Answer from the drawing. Dimensions are ordinates in mm from the lowest x, y and z of the part. A direction names the side the tool comes from. Give positions to 0.01 mm unless a question says otherwise; leave off trailing zeros. Write each loop counter-clockwise with the first axis right and the second up, starting at its lowest first coordinate (ties: lowest second). Pieces come first, ordered by that corner, then holes. Notation, with made-up numbers: (-16, -23.5) -> (42, -23.5) arc R21 cw to (42, -10.5) -> close; hole circle Ø10 at (37.25, 74.5). An arc over 180 degrees is marked (long way). Put each result on its own line as item: value. Start each with the question number.
1) Find the intervals of material crossed by line 1 along Z through (x, y) = (6.5, 4.75); line 2 along X through (y, z) = (7.5, 3.75); line 3 along Z through (x, y) = (5.5, 10.5), in increasing order. Write a range as from..to.
2) A cutting plane is placed at B-B (x = 11). Write down the section's boundary in (y, z), then the cut area to 3 significant figures.
3) For the marked faces 1, 2 and 3, determine the directions among +Z, -Z, +X, -X, +Y, -Y from which every point of the face is accessible in a straight line to the end or side of a thin tool.
4) A cutting plane is placed at D-D (x = 16.25). Write down the section's boundary in (y, z).
5) A cutting plane is placed at C-C (z = 2.25). Write down the section's boundary in (x, y), then the cut area to 3 significant figures.
6) A cutting plane is placed at A-A (y = 11). Write down the section's boundary in (x, z), then the cut area to 4 significant figures.
7) Flat-ended cylindrical pins translate along their axes: pin 1 Ø12 at (y, z) = (6, 7.5) entering from -X; pin 2 Ø3 at (y, z) = (9.5, 16.5) entering from +X; pin 3 Ø8 at (y, z) = (6.5, 6.5) entering from +X. Find the tip coordinate at first contact, or state that the pin passes through.
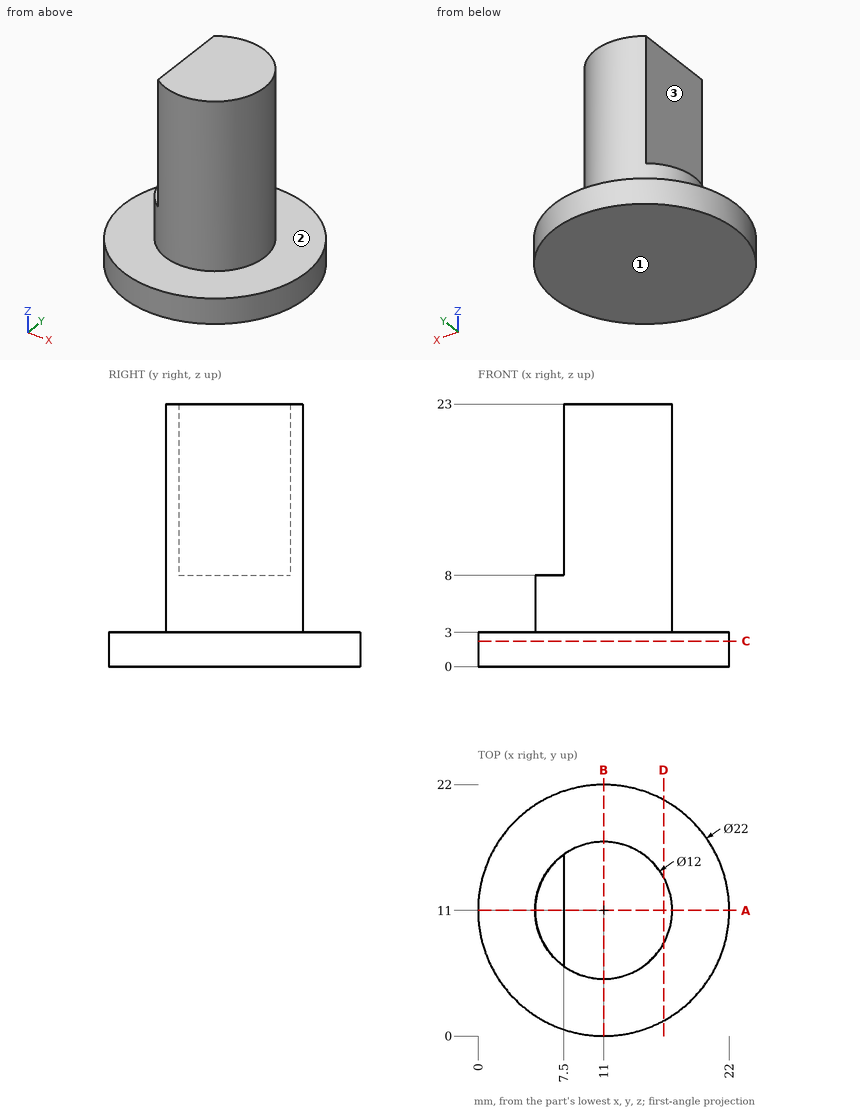
Reply:
1. line 1: z = 0..3
1. line 2: x = 6.13..15.87
1. line 3: z = 0..8
2. outline: (0, 0) -> (22, 0) -> (22, 3) -> (17, 3) -> (17, 23) -> (5, 23) -> (5, 3) -> (0, 3) -> close
2. area: 306 mm2
3. face 1: -Z, +X, -X, +Y, -Y
3. face 2: +Z
3. face 3: +Z, -X, +Y, -Y
4. outline: (1.33, 0) -> (20.67, 0) -> (20.67, 3) -> (13.9, 3) -> (13.9, 23) -> (8.1, 23) -> (8.1, 3) -> (1.33, 3) -> close
5. outline: circle Ø22 at (11, 11)
5. area: 380 mm2
6. outline: (0, 0) -> (22, 0) -> (22, 3) -> (17, 3) -> (17, 23) -> (7.5, 23) -> (7.5, 8) -> (5, 8) -> (5, 3) -> (0, 3) -> close
6. area: 268.5 mm2
7. pin 1: stops at x = 0.05
7. pin 2: stops at x = 17
7. pin 3: stops at x = 21.7
